Autodesk Inventor part; units mm, degrees
ref_plane "YZ Plane" through (0, 0, 0) normal (1, 0, 0) x (0, 1, 0)
ref_plane "XZ Plane" through (0, 0, 0) normal (0, 1, 0) x (-1, 0, 0)
ref_plane "XY Plane" through (0, 0, 0) normal (0, 0, 1) x (1, 0, 0)
sketch "Sketch1" plane through (0, 0, 0) normal (0, 0, 1) x (1, 0, 0)
  line L0 (0, 0) -> (0, 137.0131)
  line L1 (-11.7886, 12.2907) -> (-39.6863, 18.4755) construction
  line L2 (-39.6863, 18.4755) -> (-33.3297, 47.1481) construction
  line L3 (-33.3297, 47.1481) -> (-5.432, 40.9633) construction
  line L4 (-5.432, 40.9633) -> (-11.7886, 12.2907) construction
  line L5 (-39.6863, 18.4755) -> (-5.432, 40.9633) construction
  line L6 (-33.3297, 47.1481) -> (-11.7886, 12.2907) construction
  circle A0 centre (-53.975, 12.7) radius 3.175
  circle A1 centre (-53.975, 12.7) radius 9.525
  line L7 (0, 0) -> (-54.5315, 3.1913) construction
  line L8 (-62.4238, 17.0982) -> (0, 137.0131)
  line L9 (-27.1302, 45.7737) -> (-37.4529, 28.5497) construction
  line L10 (-11.6315, 42.3377) -> (-9.5552, 22.3649) construction
  line L11 (-19.3809, 44.0557) -> (-25.7374, 15.3831) construction
  line L12 (0, 104.775) -> (-15.0457, 108.1106)
  line L13 (-35.3766, 8.5768) -> (-19.8779, 5.1408) construction
  line L14 (-19.8779, 5.1408) -> (-21.2523, -1.0586) construction
  line L15 (-21.2523, -1.0586) -> (-36.751, 2.3773) construction
  line L16 (-36.751, 2.3773) -> (-35.3766, 8.5768) construction
  line L17 (-35.3766, 8.5768) -> (-44.7305, 2.6177) construction
  line L18 (-19.8779, 5.1408) -> (-17.2457, 1.0092) construction
  line L19 (-5.432, 40.9633) -> (-33.3297, 47.1481) construction
  line L20 (-33.3297, 47.1481) -> (-32.2475, 52.0296) construction
  line L21 (-32.2475, 52.0296) -> (-4.3498, 45.8448) construction
  line L22 (-4.3498, 45.8448) -> (-5.432, 40.9633) construction
  line L23 (-53.2878, 15.7997) -> (-53.975, 12.7) construction
  line L24 (-53.975, 12.7) -> (-57.0747, 13.3872) construction
  line L25 (-27.6272, 6.8588) -> (-34.4992, -24.1386) construction
  line L26 (-31.8676, 50.076) -> (-5.5198, 44.2349) construction
  line L27 (-5.5198, 44.2349) -> (-4.489, 48.8845) construction
  line L28 (-4.489, 48.8845) -> (-30.8368, 54.7256) construction
  line L29 (-30.8368, 54.7256) -> (-31.8676, 50.076) construction
  line L30 (-31.3522, 52.4008) -> (-5.0044, 46.5597) construction
  circle A2 centre (-29.0274, 51.8854) radius 1.4732 construction
  circle A3 centre (-22.8279, 50.5111) radius 1.4732 construction
  circle A4 centre (-16.6284, 49.1367) radius 1.4732
  circle A5 centre (-10.4289, 47.7623) radius 1.4732
  circle A6 centre (-7.6985, 96.7513) radius 1.4732
  line L31 (-53.975, 12.7) -> (-5.4185, 105.9762) construction
  line L32 (-31.2085, 56.4341) -> (0, 49.5153) construction
  circle A7 centre (-7.6985, 96.7513) radius 4.7625 construction
  line L33 (-4.7625, 50.5712) -> (-4.7625, 105.8308) construction
  line L34 (-26.3948, 55.3669) -> (-7.323, 92.0036) construction
  line L35 (-3.5958, 94.3328) -> (-4.7625, 94.5914) construction
  line L36 (-17.2457, 1.0092) -> (0, 1.0092) construction
  line L37 (0, 1.0092) -> (0, -2.1658) construction
  line L38 (0, -2.1658) -> (-17.2457, -2.1658) construction
  line L39 (-17.2457, -2.1658) -> (-17.2457, 1.0092) construction
  circle A8 centre (-12.7, 7.9375) radius 1.5875 construction
  line L40 (-12.7, 7.9375) -> (0, 7.9375) construction
  line L41 (0, 7.9375) -> (-17.2457, 1.0092)
  circle A9 centre (-12.7, 7.9375) radius 3.175 construction
  line L42 (-9.525, 7.9375) -> (-9.525, 4.111) construction
  line L43 (-9.525, 7.9375) -> (0, 7.9375) construction
  line L44 (-17.9187, 46.9837) -> (-16.8879, 51.6333) construction
  line L45 (-12.4942, 45.7811) -> (-26.2381, -16.2137) construction
  line L46 (0, 53.6985) -> (0, 7.9375) construction
  line L47 (-26.2381, -16.2137) -> (-20.0386, -17.5881) construction
  line L48 (-20.0386, -17.5881) -> (-8.7313, 7.9375)
  circle A10 centre (-12.7, 6.35) radius 1.4224
  line L49 (0, 13.4938) -> (-4.7625, 13.4938) construction
  line L50 (-4.7625, 13.4938) -> (-4.7625, 24.6063) construction
  line L51 (-4.7625, 24.6063) -> (0, 24.6063) construction
  line L52 (0, 24.6063) -> (0, 13.4938) construction
  line L53 (-4.7625, 19.05) -> (0, 19.05) construction
  circle A11 centre (-2.3813, 19.05) radius 1.4224
  line L54 (-20.7405, 8.5842) -> (-9.7454, 58.18) construction
  line L55 (-9.7454, 58.18) -> (-3.5459, 56.8056) construction
  line L56 (-3.5459, 56.8056) -> (-14.5411, 7.2098) construction
  line L57 (-14.5411, 7.2098) -> (-20.7405, 8.5842) construction
  line L58 (-12.7, 6.35) -> (-12.7, 7.9375) construction
  line L59 (-11.5442, 1.5875) -> (-9.525, 1.5875) construction
  line L60 (-9.525, 1.5875) -> (-9.525, 7.9375) construction
  line L61 (-9.525, 7.9375) -> (-11.5442, 7.9375) construction
  line L62 (-11.5442, 7.9375) -> (-11.5442, 1.5875) construction
  line L63 (-9.7454, 58.18) -> (-15.9449, 59.5544) construction
  line L64 (-18.8691, 53.6985) -> (0, 53.6985)
  line L65 (-9.7454, 58.18) -> (-17.3193, 53.3549) construction
  arc A12 (-10.2313, 55.9882) -> (-11.9373, 58.6659) centre (-11.0843, 57.3271) ccw construction
  line L66 (-4.7625, 57.15) -> (0, 57.15) construction
  circle A13 centre (-2.3813, 57.15) radius 1.4224
  circle A14 centre (-2.3813, 63.5) radius 1.4224
  line L67 (0, 7.9375) -> (-45.2378, 7.9375) construction
  line L68 (-45.2378, 7.9375) -> (-45.2378, -28.575) construction
  line L69 (-45.2378, -28.575) -> (0, -28.575)
  line L70 (0, -28.575) -> (0, 7.9375)
  line L71 (-45.2378, -28.575) -> (-62.6076, 8.6746)
  line L72 (-60.0032, 20.0747) -> (-18.8691, 53.6985)
  line L73 (-20.0386, -17.5881) -> (-20.0386, -28.575) construction
  line L74 (-20.2435, 47.4991) -> (-19.2127, 52.1487) construction
  line L75 (-12.7, -28.575) -> (-12.7, -1.0217)
  circle A15 centre (-23.8125, -19.05) radius 1.7526
  circle A16 centre (-15.875, -14.2875) radius 1.7526
  circle A17 centre (-23.8125, -19.05) radius 3.175 construction
  circle A18 centre (-2.3813, 69.85) radius 1.4224
  circle A19 centre (-2.3813, 76.2) radius 1.4224
  circle A20 centre (-15.875, -14.2875) radius 3.175 construction
  circle A21 centre (-46.0375, -19.05) radius 1.7526
  arc A22 (0, 104.775) -> (-15.0457, 108.1106) centre (-7.9697, 104.427) ccw
  circle A23 centre (-7.9697, 104.427) radius 1.4224
  line L76 (-7.9697, 104.427) -> (-15.0457, 108.1106) construction
  line L77 (-7.9697, 104.427) -> (0, 104.775) construction
  point P0 (-22.5591, 29.7194)
  point P1 (-20.7484, 1.2142)
  point P2 (-36.3367, 4.2458)
  point P3 (-49.5768, 21.1488)
  point P4 (-11.1125, 7.9375)
  point P5 (-11.4283, 6.9872)
  point P6 (-11.9574, 7.9375)
  point P7 (-13.9717, 6.9872)
  point P8 (-9.525, 6.1457)
  point P9 (-10.6215, 3.6705)
  dimension "d74" = 6.35
  dimension "d14" = 29.3687
  dimension "d15" = 28.575
  dimension "d16" = 12.5
  dimension "d17" = 6.35
  dimension "d19" = 53.975
  dimension "d22" = 19.05
  dimension "d23" = 7.9375
  dimension "d24" = 19.05
  dimension "d26" = 102.5
  dimension "d29" = 6.35
  dimension "d31" = 7.9375
  dimension "d34" = 5
  dimension "d35" = 26.9875
  dimension "d38" = 31.75
  dimension "d40" = 26.9875
  dimension "d41" = 4.7625
  dimension "d42" = 2.9464
  dimension "d43" = 2.3813
  dimension "d46" = 6.35
  dimension "d51" = 2.9464
  dimension "d52" = 92.075
  dimension "d53" = 6.35
  dimension "d54" = 9.525
  dimension "d55" = 4.7625
  dimension "d56" = 4.7625
  dimension "d60" = 12.7
  dimension "d61" = 3.175
  dimension "d63" = 3.175
  dimension "d66" = 3.175
  dimension "d67" = 12.7
  dimension "d72" = 8.7312
  dimension "d73" = 7.9375
  dimension "d80" = 12.7
  dimension "d82" = 7.9375
  dimension "d83" = 63.5
  dimension "d85" = 6.35
  dimension "d86" = 104.775
  dimension "d87" = 2.8448
  dimension "d88" = 4.7625
  dimension "d89" = 11.1125
  dimension "d90" = 2.8448
  dimension "d91" = 19.05
  dimension "d92" = 6.35
  dimension "d93" = 50.8
  dimension "d94" = 25.4
  dimension "d95" = 8.7312
  dimension "d96" = 9.525
  dimension "d97" = 6.35
  dimension "d99" = 6.35
  dimension "d101" = 3.175
  dimension "d106" = 2.8448
  dimension "d107" = 57.15
  dimension "d110" = 6.35
  dimension "d136" = 3.175
  dimension "d138" = 28.575
  dimension "d139" = 12.7
  dimension "d140" = 3.5052
  dimension "d141" = 3.5052
  dimension "d142" = 9.525
  dimension "d143" = 3.175
  dimension "d144" = 11.1125
  dimension "d145" = 6.35
  dimension "d146" = 14.2875
  dimension "d149" = 6.35
extrude "Extrusion1" add sketch "Sketch1" along normal blind 3.175 contours L70 L69 L75 L48 L41 L0 | L41 L48 L75 L69 L71 A1 L72 L64 L0 | L64 L72 A1 L8 L12 L0 | L12 A22 | A1
fillet "Fillet6" radius 12.7 1 edges at (-45.2378, -28.575, 1.5875)
equation "\"d56\" = d55"
properties part number "Uprights" material "UHMW, White"
Work out the finished part from the listing and answer in its coordinate system (mm). Round coordinates to 2 decimals unless told otherwise and drop trailing zeros. Write each loop counter-clockwise with the first axis right and the second up, starting at its lowest first coordinate (ties: lowest second). Pieces come first, ordered by that corner, then holes. Notation, with made-up numbers: (3.25, -11.5) - (28.25, -11.5) arc R20 ccw to (28.25, 21.5) - close; hole circle Ø3 at (46, 79.5). An arc over 180 degrees is marked (long way). Return JSON: item names as keys, results as strings. Group by question number.
Q1. The part is cut by section A-A on y = 12.7. Write down the section's boundary in (x, z) (3 decimals), then the cut area to 3 significant figures.
Q2. Find the intervals of material crossed by L1, parallel to X at y = -18.5, z = 1; L2, parallel to Y at x = -55, z = 2.9 (3 decimals); L3, parallel to X at y = 11, z = 1.4, in increasing order.
Q3. The part is cut by section C-C on y = -19.05. Write down the section's boundary in (x, z) (3 decimals), then the cut area to 3 significant figures.
Q4. The part is cut by section B-B on x = -55. Write down the section's boundary in (y, z) (3 decimals), then the cut area to 3 significant figures.
Q5. The part is cut by section D-D on z = 2.1. Count the separate pieces of the cut face and the enclosed holes in it, then the cut area to 3 significant figures.
Q6. The mould has two halves that part along X. Classify faces 1 (the cylindrical face through (-2.57, 17.64, 1.57)), 2 (the cylindrical face through (-8.155, 103.017, 1.565)), 3 (the cylindrical face through (-6.386, 112.246, 1.565)), 4 (the cylindrical face through (-44.06, -26.53, 1.61)): released by +X, released by -X, zero draft, split by the parting line, or undercut.
Q7. This flat-tipped pin is pushed along its axis until it touches: pin 1 Ø1 at (x, z) = (-42, 0.5) entering from +Y. Where does it stop, or does it pass through?
Solved:
{
 "1": {"outline": "(-63.5, 0) - (-57.15, 0) - (-57.15, 3.175) - (-63.5, 3.175) - close; (-50.8, 0) - (0, 0) - (0, 3.175) - (-50.8, 3.175) - close", "area": "181 mm²"},
 "2": {"L1": "-49.94 to -47.7, -44.37 to -25.48, -22.15 to 0", "L2": "-7.64 to 9.695, 15.705 to 31.359", "L3": "-63.35 to -56.66, -51.29 to 0"},
 "3": {"outline": "(-49.679, 0) - (-47.79, 0) - (-47.79, 3.175) - (-49.679, 3.175) - close; (-44.285, 0) - (-25.565, 0) - (-25.565, 3.175) - (-44.285, 3.175) - close; (-22.06, 0) - (0, 0) - (0, 3.175) - (-22.06, 3.175) - close", "area": "135 mm²"},
 "4": {"outline": "(-7.64, 0) - (9.695, 0) - (9.695, 3.175) - (-7.64, 3.175) - close; (15.705, 0) - (31.359, 0) - (31.359, 3.175) - (15.705, 3.175) - close", "area": "105 mm²"},
 "5": {"separate pieces": "1", "enclosed holes": "14", "area": "5,970 mm²"},
 "6": {"face 1": "undercut", "face 2": "undercut", "face 3": "split by the parting line", "face 4": "released by -X"},
 "7": {"pin 1": "y = 57.29"}
}
